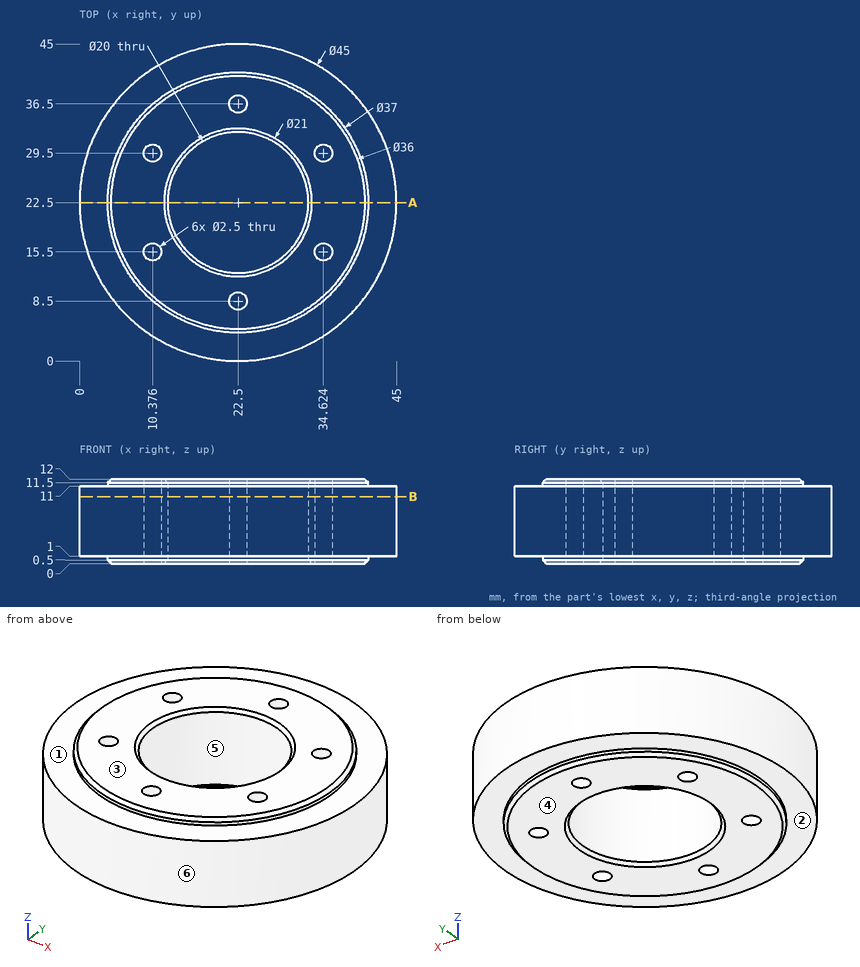
For this review, use the dimensioned drawing (mm, ordinates from the lowest corner) and the shaded views. A direction names the side the tool comes from. Round coordinates to 2 decimals unless told otherwise and drop trailing zeros. Loops run counter-clockwise (first coordinate to the right, second up) from the corner with the lowest first, then second, coordinate; pieces in that order, holes last. Notation, with made-up numbers: M 55,82.25 L 88,82.25 A5 ccw 88,91.25 Z; hole C 41,-12.75 d9. An arc over 180 degrees is marked long. Answer as CSV lines item,"result".
1. For the marked faces 1, 2 and 3, list the 3-axis set-ups (+Z, -Z, +X, -X, +Y, -Y) from which the entire face can be reached by the end or side of a thin tool; tool diameter is ignored.
Outcome:
face 1,"+Z"
face 2,"-Z"
face 3,"+Z, +X, -X, +Y, -Y"
2. We need section B-B (z = 9.5). Count the separate pieces of the cut face and the enclosed holes in it, plus the area to 3 significant figures.
Outcome:
separate pieces,"1"
enclosed holes,"7"
area,"1,250 mm2"
3. To check wall thickness, follow L1, parallel to Y at x = 22.5, z = 6.75; L2, parallel to Y at x = 9.5, z = 2.25 (1 decimal); L3, parallel to X at y = 21.5, z = 4.5. State the ranges of each line that lie inside material, in increasing order. Write a range as [from, to].
Outcome:
L1,"y = [0, 7.25], [9.75, 12.5], [32.5, 35.25], [37.75, 45]"
L2,"y = [4.1, 14.6], [16.4, 28.6], [30.4, 40.9]"
L3,"x = [0.02, 12.55], [32.45, 44.98]"
4. Insertion check: pin 1 Ø13.5 at (x, y) = (21, 24) entering from -Z; pin 2 Ø1 at (y, z) = (27, 8) entering from -X; pin 3 Ø1.5 at (y, z) = (29.5, 9) entering from +X (1 decimal); pin 4 Ø1 at (x, z) = (6.5, 5) entering from -Y. Each pin has a flat end and moves straight along its axis. Give the tip position at first contact, or say it passes through.
Outcome:
pin 1,"passes through"
pin 2,"stops at x = 0.36"
pin 3,"stops at x = 44.1"
pin 4,"stops at y = 6.19"
5. We need section A-A (y = 22.5). Give the boundary of the cut face in (x, z), plus the area to 3 significant figures.
Outcome:
outline,"M 0,1 L 4,1 L 4,0.5 L 4.5,0 L 12,0 L 12.5,0.5 L 12.5,11.5 L 12,12 L 4.5,12 L 4,11.5 L 4,11 L 0,11 Z; M 32.5,0.5 L 33,0 L 40.5,0 L 41,0.5 L 41,1 L 45,1 L 45,11 L 41,11 L 41,11.5 L 40.5,12 L 33,12 L 32.5,11.5 Z"
area,"283 mm2"
6. Draft analysis for pull direction Y (two halves, no side actions). For the marked faces 4, 5 and 6, state which applies: pulls with the +Y half, pulls with the -Y half, needs draft (parallel to the pull), parting line crosses it, or undercut.
Outcome:
face 4,"needs draft"
face 5,"undercut"
face 6,"parting line crosses it"
